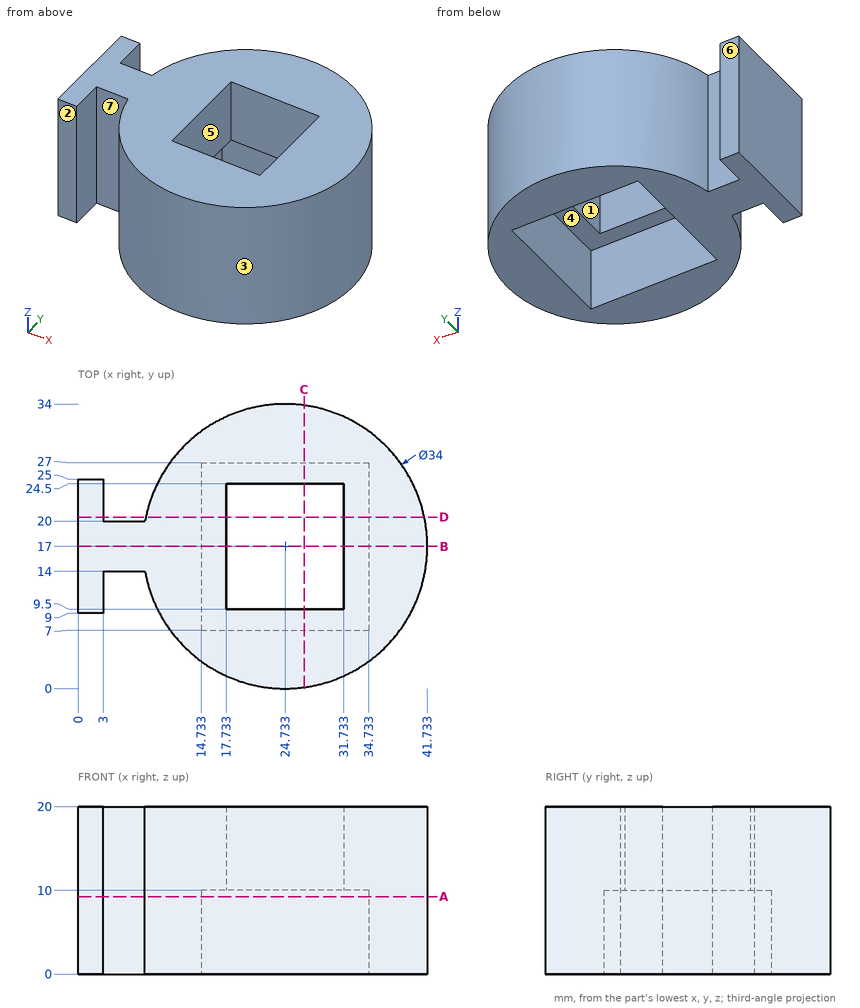
Design review of the part shown in the three views and the two pictorial views. Dimensions are in mm from the part's minimum x, y and z. A direction names the side the tool comes from. Round coordinates to 2 decimals unless told otherwise and drop trailing zeros. Loops run counter-clockwise (first coordinate to the right, second up) from the corner with the lowest first, then second, coordinate; pieces in that order, holes last. Notation, with made-up numbers: (47.5, -4) -> (86.5, -4) arc R16 cw to (86.5, 1) -> close; hole circle Ø6 at (86, 72). An arc over 180 degrees is marked (long way). Return JSON: item names as keys, results as strings.
(1) For pin 1 (10 mm diameter, centred on y = 24.5, z = 17.5, fed in from +X); pin 2 (1.5 mm diameter, centred on y = 30, z = 6, fed in from +X); pin 3 (4 mm diameter, centred on y = 11, z = 6, fed in from +X), all flat-tipped, find the tip position at first contact; note any pin that passes through.
Solved:
{"pin 1": "x = 41.55", "pin 2": "x = 36.52", "pin 3": "x = 41.26"}
(2) Add section D-D on y = 20.5. Write out the cut boundary in (x, z).
Solved:
{"outline": "(0, 0) -> (3, 0) -> (3, 20) -> (0, 20) -> close; (8.1, 0) -> (14.73, 0) -> (14.73, 10) -> (17.73, 10) -> (17.73, 20) -> (8.1, 20) -> close; (31.73, 10) -> (34.73, 10) -> (34.73, 0) -> (41.37, 0) -> (41.37, 20) -> (31.73, 20) -> close"}
(3) For the marked faces 4, 5, 6 and 7, list the 3-axis set-ups (+Z, -Z, +X, -X, +Y, -Y) from which the entire face can be reached by the end or side of a thin tool; tool diameter is ignored.
Solved:
{"face 4": "-Z", "face 5": "+Z, -Z", "face 6": "+Z, -Z, -X, +Y", "face 7": "+Z, -Z, -Y"}
(4) For line 1 (X direction, y = 11.5, z = 16); line 2 (X direction, y = 12, z = 5) (1 decimal); line 3 (Y direction, x = 4.5, z = 17.75), list the stretches that pass through material, from the lowest coordinate up.
Solved:
{"line 1": "0 to 3, 8.65 to 17.73, 31.73 to 40.82", "line 2": "0 to 3, 8.5 to 14.7, 34.7 to 41", "line 3": "14 to 20"}
(5) Add section A-A on z = 9.25. Write out the cut boundary in (x, y).
Solved:
{"outline": "(0, 9) -> (3, 9) -> (3, 14) -> (8, 14) arc R17 ccw (long way) to (8, 20) -> (3, 20) -> (3, 25) -> (0, 25) -> close; hole (14.73, 7) -> (34.73, 7) -> (34.73, 27) -> (14.73, 27) -> close"}
(6) Add section B-B on y = 17. Write out the cut boundary in (x, z), plus the area to 3 significant figures.
Solved:
{"outline": "(0, 0) -> (14.73, 0) -> (14.73, 10) -> (17.73, 10) -> (17.73, 20) -> (0, 20) -> close; (31.73, 10) -> (34.73, 10) -> (34.73, 0) -> (41.73, 0) -> (41.73, 20) -> (31.73, 20) -> close", "area": "495 mm2"}
(7) The part is to be moulded in two halves that separate along Y. For the marked faces 1, 2 and 3, say which applies: released by +Y, released by -Y, zero draft, split by the parting line, or undercut.
Solved:
{"face 1": "undercut", "face 2": "released by -Y", "face 3": "split by the parting line"}
(8) Add section C-C on x = 27. Write out the cut boundary in (y, z).
Solved:
{"outline": "(0.15, 0) -> (7, 0) -> (7, 10) -> (9.5, 10) -> (9.5, 20) -> (0.15, 20) -> close; (24.5, 10) -> (27, 10) -> (27, 0) -> (33.85, 0) -> (33.85, 20) -> (24.5, 20) -> close"}
